```python
from build123d import *

# Parameters (mm, degrees)
ESQUISSE1_W                   = 24
ESQUISSE1_H                   = 30
BOSS_EXTRU_1_DEPTH            = 20
ESQUISSE2_W                   = 12
ESQUISSE2_H                   = 4
ENL_V_MAT_EXTRU_1_DEPTH       = 31.01666204
ESQUISSE3_W                   = 12
ESQUISSE3_H                   = 4
ENL_V_MAT_EXTRU_2_DEPTH       = 31.01666204
D_POUILLE1_ANGLE              = 45
DIAM_TRE_DU_PER_AGE_8_0_8_1_D = 8
D_GAGEMENT_M31_D              = 3.242
D_GAGEMENT_M31_DEPTH          = 20
CHANFREIN1_SIZE               = 0.379
CHANFREIN2_SIZE               = 1


with BuildPart() as part:
    # Esquisse1 → Boss.-Extru.1 (new body)
    with BuildSketch(Plane(origin=(0, 10, 0), x_dir=(1, 0, 0), z_dir=(0, 1, 0))):
        with Locations((12, 0)):
            Rectangle(ESQUISSE1_W, ESQUISSE1_H)
    extrude(amount=-BOSS_EXTRU_1_DEPTH)

    # Esquisse2 → Enlèv. mat.-Extru.1 (cut, through all)
    with BuildSketch(Plane(origin=(24, 0, 0), x_dir=(0, 0, -1), z_dir=(1, 0, 0))):
        with Locations((9, -8)):
            Rectangle(ESQUISSE2_W, ESQUISSE2_H)
    extrude(amount=-ENL_V_MAT_EXTRU_1_DEPTH, mode=Mode.SUBTRACT)

    # Esquisse3 → Enlèv. mat.-Extru.2 (cut, through all)
    with BuildSketch(Plane(origin=(24, 0, 0), x_dir=(0, 0, -1), z_dir=(1, 0, 0))):
        with Locations((-9, -8)):
            Rectangle(ESQUISSE3_W, ESQUISSE3_H)
    extrude(amount=-ENL_V_MAT_EXTRU_2_DEPTH, mode=Mode.SUBTRACT)

    # Dépouille1
    d_pouille1_faces = [part.faces().sort_by_distance(p)[0] for p in [
        (12, -8, -3),
        (12, -8, 3),
    ]]
    draft(d_pouille1_faces, Plane(origin=(0, -10, 0), x_dir=(0, 0, -1), z_dir=(0, -1, 0)), D_POUILLE1_ANGLE)

    # Diamètre du perçage Ø8.0 (8)1 (through all)
    with Locations(Plane.ZY):
        with Locations((0, 0)):
            Hole(DIAM_TRE_DU_PER_AGE_8_0_8_1_D / 2)

    # Dégagement M31
    with Locations(Plane(origin=(0, 10, 0), x_dir=(1, 0, 0), z_dir=(0, 1, 0))):
        with Locations((20, -10), (4, -10), (4, 10), (20, 10)):
            Hole(D_GAGEMENT_M31_D / 2, depth=D_GAGEMENT_M31_DEPTH)

    # Chanfrein1
    chanfrein1_edges = [part.edges().sort_by_distance(p)[0] for p in [
        (21.621, 10, -10),
        (5.621, 10, -10),
        (5.621, 10, 10),
        (21.621, 10, 10),
    ]]
    chamfer(chanfrein1_edges, length=CHANFREIN1_SIZE)

    # Chanfrein2
    chanfrein2_edges = [part.edges().sort_by_distance(p)[0] for p in [
        (0, 0, 4),
        (24, 0, 4),
    ]]
    chamfer(chanfrein2_edges, length=CHANFREIN2_SIZE)


solid = part.part
```
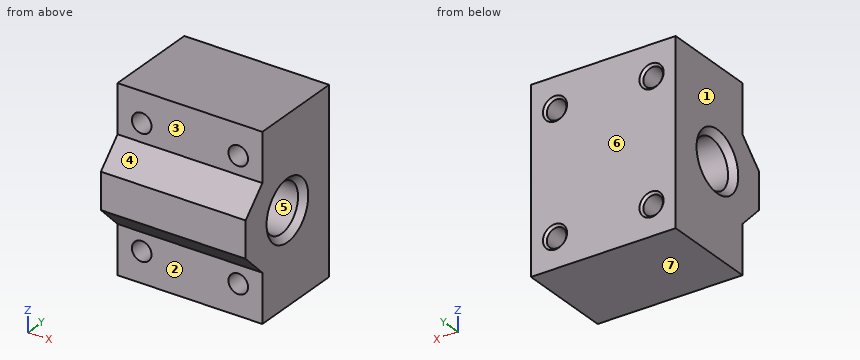
Model file for the job. Use its own axes, mm. Face numbers are marked on the shaded views. A direction names the side the tool comes from. Coordinates: 2 decimals unless noted, no trailing zeros. Order: outer loops, then holes, each group sorted by start corner. A loop starts at its lowest first (then second) coordinate and runs counter-clockwise, first axis right, second up. Notation, with made-up numbers: (45.5, 67.25) - (64.5, 67.25) arc R19 ccw to (64.5, 73.25) - close; hole circle Ø2 at (71.25, 65). An arc over 180 degrees is marked (long way). Return JSON: item names as keys, results as strings. Group by question number.
1) Mould opens along Y. For the marked faces 4, 5, 6 and 7 say: released by +Y, released by -Y, zero draft, split by the parting line, or undercut.
2) Saw through at C-C, the plane z = -10. Write the cut outline in (x, y).
3) Flat gauge pins, fed straight in: P1, Ø10, axis at y = -3.5, z = -5.5, coming from the -X side; P2, Ø1.5, axis at y = 3, z = 2, coming from the -X side; P3, Ø4, axis at x = 12.5, z = 11.5, coming from the -Y side; P4, Ø3.5, axis at x = 20, z = -10, coming from the +Y side. Where does each tip first touch, or does it go through?
4) Saw through at D-D, the plane y = 7.25. Write the cut outline in (x, z), plus the area to 3 significant figures.
5) Probe line 1 (X direction, y = -2.5, z = 10); line 2 (Z direction, x = 20, y = 5); line 3 (Y direction, x = 2.5, z = 0.25). List the from-to ranges inside material, lowest first. Write a range as from..to.
6) Tool access for the marked faces 1, 2 and 3: list every direction of +Z, -Z, +X, -X, +Y, -Y with a clear straight run to the whole face (end or side of a thin tool).
7) Saw through at B-B, the plane y = 0. Write the cut outline in (x, z), plus the area to 3 significant figures.
8) Saw through at A-A, the plane x = 4. Write the cut outline in (y, z), plus the area to 3 significant figures.
Values found:
{
 "1": {"face 4": "released by -Y", "face 5": "undercut", "face 6": "released by +Y", "face 7": "zero draft"},
 "2": {"outline": "(0, -6) - (2.38, -6) - (2.38, 9.62) - (2, 10) - (0, 10) - close; (5.62, -6) - (18.38, -6) - (18.38, 9.62) - (18, 10) - (6, 10) - (5.62, 9.62) - close; (21.62, -6) - (24, -6) - (24, 10) - (22, 10) - (21.62, 9.62) - close"},
 "3": {"P1": "stops at x = 0", "P2": "stops at x = 0.64", "P3": "stops at y = -6", "P4": "stops at y = 9.75"},
 "4": {"outline": "(0, -15) - (24, -15) - (24, 15) - (0, 15) - close; hole circle Ø3.24 at (4, -10); hole circle Ø3.24 at (4, 10); hole circle Ø3.24 at (20, -10); hole circle Ø3.24 at (20, 10)", "area": "687 mm²"},
 "5": {"line 1": "x = 0..2.38, 5.62..18.38, 21.62..24", "line 2": "z = -15..-11.62, -8.38..8.38, 11.62..15", "line 3": "y = -10..-3.99, 3.99..10"},
 "6": {"face 1": "+Z, -Z, -X, +Y, -Y", "face 2": "-Z, +X, -X, -Y", "face 3": "+Z, +X, -X, -Y"},
 "7": {"outline": "(0, -15) - (24, -15) - (24, -5) - (23, -4) - (1, -4) - (0, -5) - close; (0, 5) - (1, 4) - (23, 4) - (24, 5) - (24, 15) - (0, 15) - close; hole circle Ø3.24 at (4, -10); hole circle Ø3.24 at (4, 10); hole circle Ø3.24 at (20, -10); hole circle Ø3.24 at (20, 10)", "area": "493 mm²"},
 "8": {"outline": "(-10, -3) - (-6, -7) - (-6, -8.38) - (9.62, -8.38) - (10, -8) - (10, 8) - (9.62, 8.38) - (-6, 8.38) - (-6, 7) - (-10, 3) - close; (-6, -15) - (10, -15) - (10, -12) - (9.62, -11.62) - (-6, -11.62) - close; (-6, 11.62) - (9.62, 11.62) - (10, 12) - (10, 15) - (-6, 15) - close; hole circle Ø8 at (0, 0)", "area": "366 mm²"}
}
